Here's how the part is built. I have some questions about the finished solid (model axes, mm). A direction names the side the tool comes from. Round coordinates to 2 decimals unless told otherwise and drop trailing zeros. Loops run counter-clockwise (first coordinate to the right, second up) from the corner with the lowest first, then second, coordinate; pieces in that order, holes last. Notation, with made-up numbers: (15.25, 69) - (61.25, 69) arc R21 cw to (61.25, 80) - close; hole circle Ø11 at (-32, 28). An arc over 180 degrees is marked (long way). Answer as a JSON object with one key per item and string values. Group by question number.
1) I want a section at D-D, the plane z = -10.5. Please give me the cut outline in (x, y), then the cut area to 3 significant figures.
2) I want a section at C-C, the plane y = 0.8. Please give me the cut outline in (x, z).
3) If we mould it in two halves opening along Z, with no side actions, what happens to faces 5 (the face through (0, -1, -23)), 6 (the face through (-0.2, 0, 8.3)), 7 (the face through (-10, -1, -16))? For each: pulls with the +Z half, pulls with the -Z half, needs draft (parallel to the pull), parting line crosses it, or undercut.
4) I want a section at A-A, the plane x = 0.5. Please give me the cut outline in (y, z), then the cut area to 3 significant figures.
5) Will these pins go through, and if not, where does the flat tip stop? P1, Ø9.5, axis at x = 3.5, z = 2.5, coming from the -Y side; P2, Ø1.8, axis at y = 0, z = -19.5, coming from the +X side; P3, Ø1, axis at x = -1.5, y = 1, coming from the -Z side; P4, Ø0.8, axis at x = 10.5, y = 1.5, coming from the +Z side.
6) I want a section at B-B, the plane z = -5.5. Please give me the cut outline in (x, y).
7) Which directions (+Z, -Z, +X, -X, +Y, -Y) give clear straight access to the entire face, cutting with the end or side of a thin tool? Please do faces 1 (the face through (0, 1, -11.5)), 2 (the face through (0, 1, -8)), 3 (the face through (0, -1, -9.5)), 4 (the face through (10, -1, -16)).
8) If I drill on line 1 along Z through (x, y) = (-2.5, 1.3); line 2 along Z through (x, y) = (-8.5, -1.05); line 3 along X through (y, z) = (0.6, 7.5), over which ranges is the centre line in solid material (lowest first)? Write a range as [from, to].
from build123d import *

# Parameters (mm, degrees)
SKETCH1_W             = 23
SKETCH1_H             = 19
SKETCH1_W_2           = 20
SKETCH1_H_2           = 16
BOSS_EXTRUDE1_DEPTH   = 2
SKETCH2_W             = 20
SKETCH2_H             = 13.5
BOSS_EXTRUDE3_DEPTH   = 1.5
BOSS_EXTRUDE3_2_DEPTH = 1.5
SKETCH3_W             = 20
SKETCH3_H             = 2
BOSS_EXTRUDE4_DEPTH   = 2


with BuildPart() as part:
    # Sketch1 → Boss-Extrude1 (new body)
    with BuildSketch(Plane(origin=(0, 0, 0), x_dir=(1, 0, 0), z_dir=(0, 1, 0))):
        Rectangle(SKETCH1_W, SKETCH1_H)
        Rectangle(SKETCH1_W_2, SKETCH1_H_2, mode=Mode.SUBTRACT)
    extrude(amount=BOSS_EXTRUDE1_DEPTH)



with BuildPart() as body_2:
    # Sketch2 → Boss-Extrude3 (new body)
    with BuildSketch(Plane.XZ):
        with Locations((0, 16.25)):
            Rectangle(SKETCH2_W, SKETCH2_H)
    extrude(amount=BOSS_EXTRUDE3_DEPTH)


with BuildPart() as body_3:
    # Sketch2 → Boss-Extrude3 2 (new body)
    with BuildSketch(Plane.XZ):
        with Locations((0, -16.25)):
            Rectangle(SKETCH2_W, SKETCH2_H)
    extrude(amount=BOSS_EXTRUDE3_2_DEPTH)


with BuildPart() as part_1:
    add(part.part)

    add(body_2.part)  # Boss-Extrude4 merges body 2

    add(body_3.part)  # Boss-Extrude4 merges body 3
    # Sketch3 → Boss-Extrude4 (add)
    with BuildSketch(Plane(origin=(0, 0, 0), x_dir=(1, 0, 0), z_dir=(0, 1, 0))):
        with Locations((0, 10.5)):
            Rectangle(SKETCH3_W, SKETCH3_H)
        with Locations((0, -10.5)):
            Rectangle(SKETCH3_W, SKETCH3_H)
    extrude(amount=BOSS_EXTRUDE4_DEPTH)


solid = part_1.part
Outcome:
{
 "1": {"outline": "(-10, -1.5) - (10, -1.5) - (10, 2) - (-10, 2) - close", "area": "70.0 mm^2"},
 "2": {"outline": "(-11.5, -9.5) - (-10, -9.5) - (-10, -11.5) - (10, -11.5) - (10, -9.5) - (11.5, -9.5) - (11.5, 9.5) - (10, 9.5) - (10, 11.5) - (-10, 11.5) - (-10, 9.5) - (-11.5, 9.5) - close; hole (-10, -8) - (10, -8) - (10, 8) - (-10, 8) - close"},
 "3": {"face 5": "pulls with the -Z half", "face 6": "undercut", "face 7": "needs draft"},
 "4": {"outline": "(-1.5, -23) - (0, -23) - (0, -11.5) - (2, -11.5) - (2, -8) - (0, -8) - (0, -9.5) - (-1.5, -9.5) - close; (-1.5, 9.5) - (0, 9.5) - (0, 8) - (2, 8) - (2, 11.5) - (0, 11.5) - (0, 23) - (-1.5, 23) - close", "area": "54.5 mm^2"},
 "5": {"P1": "through", "P2": "x = 10", "P3": "z = -11.5", "P4": "z = 9.5"},
 "6": {"outline": "(-11.5, 0) - (-10, 0) - (-10, 2) - (-11.5, 2) - close; (10, 0) - (11.5, 0) - (11.5, 2) - (10, 2) - close"},
 "7": {"face 1": "-Z, +X, -X, +Y", "face 2": "+Y, -Y", "face 3": "+X, -X, -Y", "face 4": "-Z, +X, +Y, -Y"},
 "8": {"line 1": "[-11.5, -8], [8, 11.5]", "line 2": "[-23, -9.5], [9.5, 23]", "line 3": "[-11.5, -10], [10, 11.5]"}
}
